Work out the finished part from the listing and answer in its coordinate system (mm). Face numbers are marked on the shaded views. A direction names the side the tool comes from. Coordinates: 2 decimals unless noted, no trailing zeros. Write each loop counter-clockwise with the first axis right and the second up, starting at its lowest first coordinate (ties: lowest second). Pieces come first, ordered by that corner, then holes. Notation, with made-up numbers: (50, 51) - (93, 51) arc R24 ccw to (93, 84) - close; hole circle Ø7 at (-2.5, 0). An arc over 180 degrees is marked (long way). Use CSV: the item, a comma, the result in double quotes. Start each with the question number.
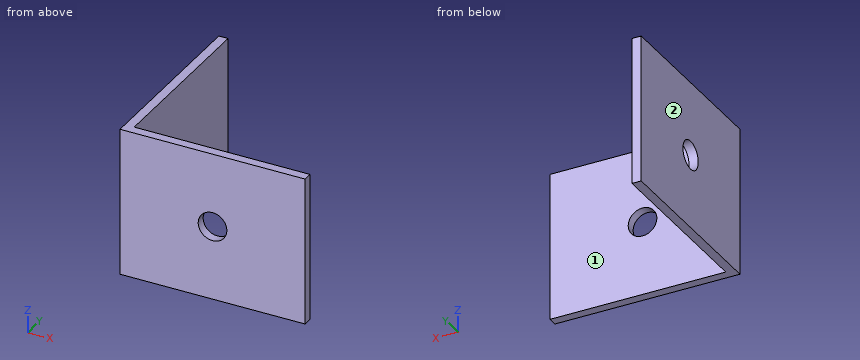
from build123d import *

# Parameters (mm, degrees)
BOSS_EXTRUDE1_DEPTH          = 25.4
F_10_0_1935_DIAMETER_HOLE1_D = 4.9149
F_10_0_1935_DIAMETER_HOLE2_D = 4.9149


with BuildPart() as part:
    # Sketch1 → Boss-Extrude1 (new body)
    with BuildSketch(Plane.XY):
        Polygon((0, 0), (0, 31.75), (1.5875, 31.75), (1.5875, 1.5875), (31.75, 1.5875), (31.75, 0), align=None)
    extrude(amount=BOSS_EXTRUDE1_DEPTH)

    # #10 (0.1935) Diameter Hole1 (through all)
    with Locations(Plane(origin=(0, 0, 0), x_dir=(-1, 0, 0), z_dir=(0, -1, 0))):
        with Locations((-15.875, -12.7)):
            Hole(F_10_0_1935_DIAMETER_HOLE1_D / 2)

    # #10 (0.1935) Diameter Hole2 (through all)
    with Locations(Plane.ZY):
        with Locations((12.7, 15.875)):
            Hole(F_10_0_1935_DIAMETER_HOLE2_D / 2)


solid = part.part
Item 1: A cutting plane is placed at B-B (x = 14.5). Determine the outline of the cut face in (y, z), then the cut area to 3 significant figures.
Item 2: Straight lines are drawn through the part: probe 1 along Y at (x, z) = (1.2, 12.7); probe 2 along Y at (x, z) = (16, 1.5). For each, find the intervals that lie inside material, in ascending order. Write a range as [from, to].
Item 3: A cutting plane is placed at C-C (y = 30). Determine the outline of the cut face in (x, z).
Item 4: Which of the six approach directions +Z, -Z, +X, -X, +Y, -Y give full straight-line access (tool end or side, diameter ignored) to the marked faces 1 and 2?
Item 5: Each of these flat-tipped pins is pushed along its axis until it touches: pin 1 (8 mm diameter, centred on y = 20.5, z = 15.5, fed in from +X); pin 2 (2 mm diameter, centred on x = 19.5, z = 14, fed in from +Y). Where does it stop, or does it pass through?
Item 6: A cutting plane is placed at A-A (z = 12.7). Determine the outline of the cut face in (x, y).
Calculated:
1,outline,"(0, 0) - (1.59, 0) - (1.59, 10.66) - (0, 10.66) - close; (0, 14.74) - (1.59, 14.74) - (1.59, 25.4) - (0, 25.4) - close"
1,area,"33.9 mm²"
2,probe 1,"y = [0, 13.42], [18.33, 31.75]"
2,probe 2,"y = [0, 1.59]"
3,outline,"(0, 0) - (1.59, 0) - (1.59, 25.4) - (0, 25.4) - close"
4,face 1,"+Z, -Z, +X, +Y"
4,face 2,"+Z, -Z, -X, +Y, -Y"
5,pin 1,"stops at x = 1.59"
5,pin 2,"stops at y = 1.59"
6,outline,"(0, 0) - (13.42, 0) - (13.42, 1.59) - (1.59, 1.59) - (1.59, 13.42) - (0, 13.42) - close; (0, 18.33) - (1.59, 18.33) - (1.59, 31.75) - (0, 31.75) - close; (18.33, 0) - (31.75, 0) - (31.75, 1.59) - (18.33, 1.59) - close"
